Answer from the drawing. Dimensions are ordinates in mm from the lowest x, y and z of the part. Give positions to 0.01 mm unless a question says otherwise; leave off trailing zeros. Order: outer loops, then holes, each group sorted by start corner. A loop starts at its lowest first (then second) coordinate and runs counter-clockwise, first axis right, second up. Notation, with made-up numbers: (-39, -26.5) -> (11, -26.5) arc R16 cw to (11, -18.5) -> close; hole circle Ø11 at (12.25, 22). An arc over 180 degrees is marked (long way). Answer as a JSON object with one key per item and string values. Group by question number.
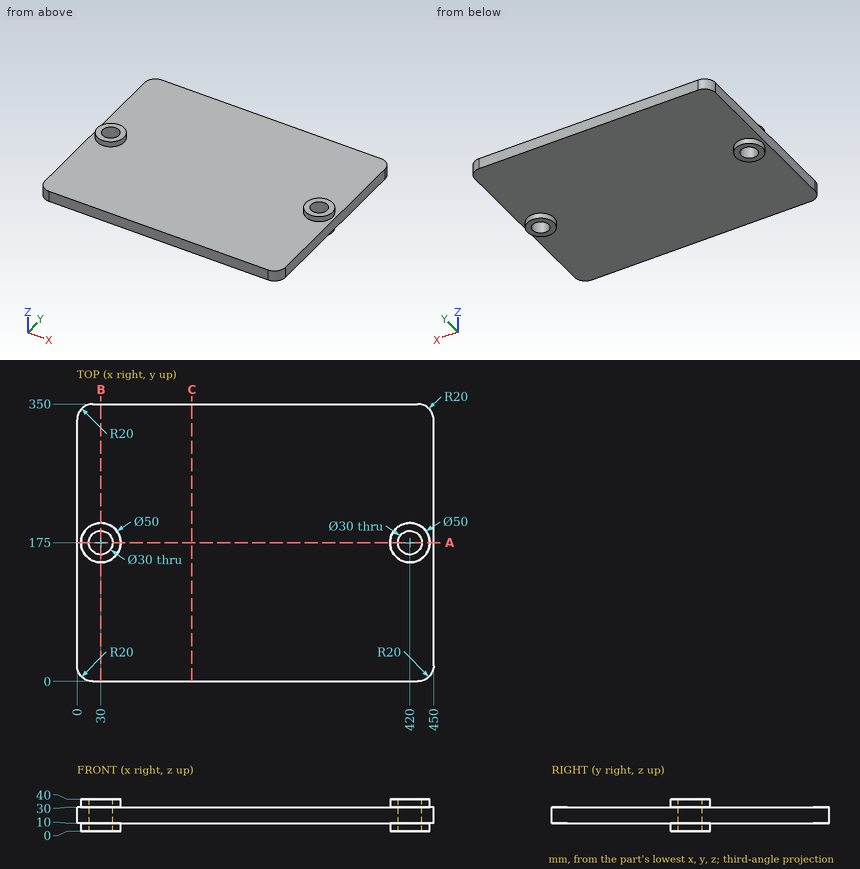
(1) A cutting plane is placed at A-A (y = 175). Determine the outline of the cut face in (x, z).
(2) Find the intervals of material crossed by line 1 along Y through (x, z) = (30, 27.5); line 2 along Z through (x, y) = (290.5, 131.5); line 3 along X through (y, z) = (188, 8), in increasing order. Write a range as [from, to].
(3) A cutting plane is placed at B-B (x = 30). Determine the outline of the cut face in (y, z).
(4) A cutting plane is placed at C-C (x = 145). Determine the outline of the cut face in (y, z), and give its area (3 significant figures).
(5) Flat-ended cylindrical pins translate along their axes: pin 1 Ø4 at (x, y) = (191.5, 111.5) entering from +Z; pin 2 Ø12 at (x, y) = (358, 284) entering from -Z. Find the tip coordinate at first contact, or state that the pin passes through.
Check sheet entries:
{
 "1": {"outline": "(0, 10) -> (5, 10) -> (5, 0) -> (15, 0) -> (15, 40) -> (5, 40) -> (5, 30) -> (0, 30) -> close; (45, 0) -> (55, 0) -> (55, 10) -> (395, 10) -> (395, 0) -> (405, 0) -> (405, 40) -> (395, 40) -> (395, 30) -> (55, 30) -> (55, 40) -> (45, 40) -> close; (435, 0) -> (445, 0) -> (445, 10) -> (450, 10) -> (450, 30) -> (445, 30) -> (445, 40) -> (435, 40) -> close"},
 "2": {"line 1": "y = [0, 160], [190, 350]", "line 2": "z = [10, 30]", "line 3": "x = [8.65, 22.52], [37.48, 51.35], [398.65, 412.52], [427.48, 441.35]"},
 "3": {"outline": "(0, 10) -> (150, 10) -> (150, 0) -> (160, 0) -> (160, 40) -> (150, 40) -> (150, 30) -> (0, 30) -> close; (190, 0) -> (200, 0) -> (200, 10) -> (350, 10) -> (350, 30) -> (200, 30) -> (200, 40) -> (190, 40) -> close"},
 "4": {"outline": "(0, 10) -> (350, 10) -> (350, 30) -> (0, 30) -> close", "area": "7,000 mm2"},
 "5": {"pin 1": "stops at z = 30", "pin 2": "stops at z = 10"}
}
